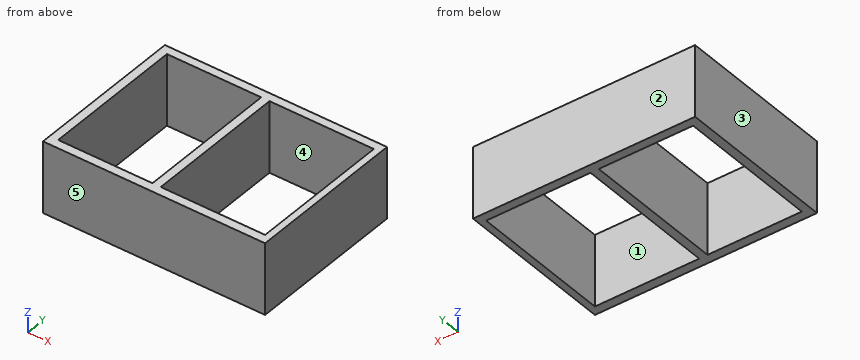
from build123d import *

# Parameters (mm, degrees)
F0_W     = 3.581136
F0_H     = 76.146152
F0_W_2   = 4.429294
F1_DEPTH = 38.1


with BuildPart() as f1:
    # F0 (on Top) → F1 (new body)
    with BuildSketch(Plane.XY):
        Polygon((-50.32431, 39.298199), (-54.847848, 39.298199), (-54.847848, -41.559964), (-50.32431, -41.559964), (-50.32431, -36.847953), align=None)
        with Locations((61.915867, 1.225123)):
            Rectangle(F0_W, F0_H)
        Polygon((63.706435, -41.559964), (63.706435, -36.847953), (60.125299, -36.847953), (4.429294, -36.847953), (0, -36.847953), (-50.32431, -36.847953), (-50.32431, -41.559964), align=None)
        with Locations((2.214647, 1.225123)):
            Rectangle(F0_W_2, F0_H)
        Polygon((63.706435, 43.821733), (-54.847848, 43.821733), (-54.847848, 39.298199), (-50.32431, 39.298199), (0, 39.298199), (4.429294, 39.298199), (60.125299, 39.298199), (63.706435, 39.298199), align=None)
    extrude(amount=F1_DEPTH)


solid = f1.part
Geometry check sheet. Reference: the model listing, model coordinates, mm. Face numbers are marked on the shaded views. A direction names the side the tool comes from. Give positions to 0.01 mm unless a question says otherwise; leave off trailing zeros. Write each loop counter-clockwise with the first axis right and the second up, starting at its lowest first coordinate (ties: lowest second). Pieces come first, ordered by that corner, then holes.
1) Set-up check for the marked faces 1 and 2: record each of +Z, -Z, +X, -X, +Y, -Y from which the full face is reachable in a straight line by a thin tool's end or side.
Values follow:
face 1: +Z, -Z
face 2: +Z, -Z, +X, -X, +Y
2) Cross-section at C-C (y = -15). Record the boundary of the cut face in (x, z), plus the area to 3 significant figures.
Values follow:
outline: (-54.85, 0) - (-50.32, 0) - (-50.32, 38.1) - (-54.85, 38.1) - close; (0, 0) - (4.43, 0) - (4.43, 38.1) - (0, 38.1) - close; (60.13, 0) - (63.71, 0) - (63.71, 38.1) - (60.13, 38.1) - close
area: 478 mm2
3) Cross-section at A-A (z = 29). Record the boundary of the cut face in (x, y).
Values follow:
outline: (-54.85, -41.56) - (63.71, -41.56) - (63.71, 43.82) - (-54.85, 43.82) - close; hole (-50.32, -36.85) - (0, -36.85) - (0, 39.3) - (-50.32, 39.3) - close; hole (4.43, -36.85) - (60.13, -36.85) - (60.13, 39.3) - (4.43, 39.3) - close
4) Release check for a two-part mould opening along X. For the marked faces 3, 4 and 5 record: released by +X, released by -X, zero draft, split by the parting line, or undercut.
Values follow:
face 3: released by -X
face 4: undercut
face 5: zero draft
5) Cross-section at B-B (x = 37.5). Record the boundary of the cut face in (y, z), plus the area to 3 significant figures.
Values follow:
outline: (-41.56, 0) - (-36.85, 0) - (-36.85, 38.1) - (-41.56, 38.1) - close; (39.3, 0) - (43.82, 0) - (43.82, 38.1) - (39.3, 38.1) - close
area: 352 mm2
6) Go/stop test with a flat-tipped pin: pin 1 Ø10 at (x, y) = (-21, -29.5) entering from -Z. Record where the tip stops, or that it passes through.
Values follow:
pin 1: passes through
7) Thickness scan on line 1 (X direction, y = -6, z = 3); line 2 (Y direction, x = -23.5, z = 21). Record the ranges inside material, lowest first.
Values follow:
line 1: x = -54.85 to -50.32, 0 to 4.43, 60.13 to 63.71
line 2: y = -41.56 to -36.85, 39.3 to 43.82
